Source: CAD feature listing. Evaluate the final solid. Frame: model axes, mm. A direction names the side the tool comes from. Give positions to 0.01 mm unless a question says otherwise; leave off trailing zeros. Loops run counter-clockwise (first coordinate to the right, second up) from the corner with the lowest first, then second, coordinate; pieces in that order, holes last.
```python
from build123d import *

# Parameters (mm, degrees)
SKETCH083_R         = 27
SKETCH083_R_2       = 3.1
PAD050_DEPTH        = 8
HOLE003_D           = 4.5
HOLE003_CSINK_D     = 9
HOLE003_CSINK_ANGLE = 90
SKETCH080_R         = 4
PAD051_DEPTH        = 1
PAD052_DEPTH        = 7
SKETCH081_R         = 1.7272
POCKET026_DEPTH     = 8.001


with BuildPart() as part:
    # Sketch083 → Pad050 (new body)
    with BuildSketch(Plane.XY):
        Circle(SKETCH083_R)
        Circle(SKETCH083_R_2, mode=Mode.SUBTRACT)
    extrude(amount=PAD050_DEPTH)

    # Hole003 (through all)
    with Locations(Plane.XY.offset(8)):
        with Locations((-8, 8), (8, 8), (8, -8), (-8, -8)):
            CounterSinkHole(HOLE003_D / 2, HOLE003_CSINK_D / 2, counter_sink_angle=HOLE003_CSINK_ANGLE)

    # Sketch080 → Pad051 (join)
    with BuildSketch(Plane.XY.offset(4.5)):
        Circle(SKETCH080_R)
    extrude(amount=PAD051_DEPTH)

    # Sketch085 → Pad052 (join)
    with BuildSketch(Plane.XY.offset(1)):
        with BuildLine():
            Line((-27, 0), (-27, 28))
            Line((-27, 28), (27, 28))
            Line((27, 28), (27, 0))
            Line((27, 0), (25, 0))
            ThreePointArc((25, 0), (0, 25), (-25, 0))
            Line((-25, 0), (-27, 0))
        make_face()
    extrude(amount=PAD052_DEPTH)

    # Sketch081 → Pocket026 (cut, through all)
    with BuildSketch(Plane.XY):
        with Locations((-18, 18)):
            Circle(SKETCH081_R)
        with Locations((17, 18)):
            Circle(SKETCH081_R)
    extrude(amount=POCKET026_DEPTH, mode=Mode.SUBTRACT)


solid = part.part
```
(1) Reachability of faces 1 (the flat face through (0.1, 27.5, 1)), 2 (the cylindrical face through (1.43, -2.75, 2.22)), 3 (the cylindrical face through (1.43, -2.75, 6.73)) from +Z, -Z, +X, -X, +Y, -Y: full face, straight path, thin tool, end or side. Return the list, or none.
A:
face 1: -Z, +Y
face 2: -Z
face 3: +Z
(2) Section D-D, the plane x = 8. Return the cut outline in (y, z), then the cut area to 3 significant figures.
A:
outline: (-25.79, 0) - (-10.25, 0) - (-10.25, 5.75) - (-12.5, 8) - (-25.79, 8) - close; (-5.75, 0) - (5.75, 0) - (5.75, 5.75) - (3.5, 8) - (-3.5, 8) - (-5.75, 5.75) - close; (10.25, 0) - (25.79, 0) - (25.79, 1) - (28, 1) - (28, 8) - (12.5, 8) - (10.25, 5.75) - close
area: 346 mm2
(3) Section C-C, the plane x = 0. Return the cut outline in (y, z).
A:
outline: (-27, 0) - (-3.1, 0) - (-3.1, 4.5) - (3.1, 4.5) - (3.1, 0) - (27, 0) - (27, 1) - (28, 1) - (28, 8) - (3.1, 8) - (3.1, 5.5) - (-3.1, 5.5) - (-3.1, 8) - (-27, 8) - close
(4) Mould query, pull axis X, two halves, no side actions, for faces 4 (the flat face through (0, 28, 4)), 5 (the flat face through (27, 14, 4)), 6 (the cylindrical face through (-6.34, -6.48, 2.83)). Classes: pulls with the +X half, pulls with the -X half, needs draft (parallel to the pull), parting line crosses it, or undercut.
A:
face 4: needs draft
face 5: pulls with the +X half
face 6: undercut
(5) First-contact query: pin 1 (5 mm diameter, centred on x = 8, y = 8, fed in from +Z); pin 2 (6 mm diameter, centred on x = -8, y = -8, fed in from +Z); pin 3 (1.5 mm diameter, centred on y = -5.5, z = 1.5, fed in from -X). Flat tips, straight axial feed; report the tip coordinate or a pass-through.
A:
pin 1: stops at z = 6
pin 2: stops at z = 6.5
pin 3: stops at x = -26.58
(6) Section B-B, the plane y = 8. Return the cut outline in (x, z), then the cut area to 3 significant figures.
A:
outline: (-27, 1) - (-25.79, 1) - (-25.79, 0) - (-10.25, 0) - (-10.25, 5.75) - (-12.5, 8) - (-27, 8) - close; (-5.75, 0) - (5.75, 0) - (5.75, 5.75) - (3.5, 8) - (-3.5, 8) - (-5.75, 5.75) - close; (10.25, 0) - (25.79, 0) - (25.79, 1) - (27, 1) - (27, 8) - (12.5, 8) - (10.25, 5.75) - close
area: 347 mm2
(7) Ray query, line 1 along X through (y, z) = (18, 5.5); line 2 along X through (y, z) = (8, 3.95); line 3 along Y through (x, z) = (-8, 2.85). Return the intervals inside material, ascending.
A:
line 1: x = -27 to -19.73, -16.27 to 15.27, 18.73 to 27
line 2: x = -27 to -10.25, -5.75 to 5.75, 10.25 to 27
line 3: y = -25.79 to -10.25, -5.75 to 5.75, 10.25 to 28
(8) Section A-A, the plane z = 3. Return the cut outline in (x, y).
A:
outline: (-27, 0) arc R27 ccw to (27, 0) - (27, 28) - (-27, 28) - close; hole circle Ø3.45 at (-18, 18); hole circle Ø4.5 at (-8, -8); hole circle Ø4.5 at (-8, 8); hole circle Ø6.2 at (0, 0); hole circle Ø4.5 at (8, -8); hole circle Ø4.5 at (8, 8); hole circle Ø3.45 at (17, 18)
